Here's how the part is built. I have some questions about the finished solid (model axes, mm). A direction names the side the tool comes from. Give positions to 0.01 mm unless a question says otherwise; leave off trailing zeros. Loops run counter-clockwise (first coordinate to the right, second up) from the corner with the lowest first, then second, coordinate; pieces in that order, holes last.
Q1. If we section it at B-B (x = 10.5): Please give me the cut outline in (y, z), plus the area to 3 significant figures.
Q2. If we section it at C-C (z = 9): Please give me the cut outline in (x, y).
Q3. We'd pull the mould along Z, two halves only. Please class faces 4 (the face through (-13, 10, -28)), 5 (the face through (0.506, 9.86, 22.994)), 6 (the face through (13, 10, -19)): +Z half, -Z half, draft (parallel to the pull), parting line (faces both ways), or undercut.
Q4. I need wall thicknesses on line 1 (Y direction, x = -9.75, z = -22); line 2 (Z direction, x = 13, y = 11.75); line 3 (Z direction, x = -14, y = 8). Which ranges of each line are inside material? Lowest first, please.
Q5. If we section it at A-A (y = 10): Please give me the cut outline in (x, z).
Q6. Will these pins go through, and if not, where does the flat tip stop? P1, Ø3, axis at x = -0.5, y = 2, coming from the -Z side; P2, Ø4, axis at y = 4.5, z = 12, coming from the +X side; P3, Ø3, axis at x = -16, y = 9.5, coming from the +Z side; P4, Ø5, axis at y = 10, z = -22, coming from the +X side.
Q7. For faces 1 (the face through (-13, 7.5, -24.3)), 2 (the face through (-0.756, 9.86, 17.984)), 3 (the face through (-2.5, 9.9, -25.2)), which set-ups out of +Z, -Z, +X, -X, +Y, -Y let a thin tool reach every point of the face, with its end or its side?
Q8. If we section it at D-D (y = 18.25): Please give me the cut outline in (x, z), plus the area to 3 significant figures.
from build123d import *

# Parameters (mm, degrees)
BOSS_EXTRU_1_DEPTH      = 20
ESQUISSE2_R             = 3
ENL_V_MAT_EXTRU_1_DEPTH = 47
ENL_V_MAT_EXTRU_2_DEPTH = 10


with BuildPart() as part:
    # Esquisse1 → Boss.-Extru.1 (new body)
    with BuildSketch(Plane(origin=(0, 0, 0), x_dir=(1, 0, 0), z_dir=(0, 1, 0))):
        with BuildLine():
            Line((-23, 0), (-23, 28))
            Line((-23, 28), (-2.5, 28))
            Line((-2.5, 28), (-2.5, 17.82554347))
            ThreePointArc((-2.5, 17.82554347), (0, -18), (2.5, 17.82554347))
            Line((2.5, 17.82554347), (2.5, 28))
            Line((2.5, 28), (23, 28))
            Line((23, 28), (23, 0))
            ThreePointArc((23, 0), (0, -23), (-23, 0))
        make_face()
    extrude(amount=BOSS_EXTRU_1_DEPTH)

    # Esquisse2 → Enlèv. mat.-Extru.1 (cut, through all)
    with BuildSketch(Plane(origin=(23, 0, 0), x_dir=(0, 0, -1), z_dir=(1, 0, 0))):
        with Locations((22, 10)):
            Circle(ESQUISSE2_R)
    extrude(amount=-ENL_V_MAT_EXTRU_1_DEPTH, mode=Mode.SUBTRACT)

    # Esquisse3 → Enlèv. mat.-Extru.2 (cut)
    with BuildSketch(Plane.ZY.offset(23)):
        Polygon((-22, 4.226497308), (-17, 7.113248654), (-17, 12.886751346), (-22, 15.773502692), (-27, 12.886751346), (-27, 7.113248654), align=None)
    extrude(amount=-ENL_V_MAT_EXTRU_2_DEPTH, mode=Mode.SUBTRACT)


solid = part.part
Check sheet entries:
1. outline: (0, -28) - (20, -28) - (20, -14.62) - (0, -14.62) - close; (0, 14.62) - (20, 14.62) - (20, 20.46) - (0, 20.46) - close; hole circle Ø6 at (10, -22)
1. area: 356 mm2
2. outline: (-21.17, 0) - (-15.59, 0) - (-15.59, 20) - (-21.17, 20) - close; (15.59, 0) - (21.17, 0) - (21.17, 20) - (15.59, 20) - close
3. face 4: -Z half
3. face 5: +Z half
3. face 6: undercut
4. line 1: y = 0 to 7, 13 to 20
4. line 2: z = -28 to -24.44, -19.56 to -12.45, 12.45 to 18.97
4. line 3: z = -28 to -27, -17 to -11.31, 11.31 to 18.25
5. outline: (-23, -28) - (-2.5, -28) - (-2.5, -25) - (-13, -25) - (-13, -27) - (-23, -27) - close; (-23, -17) - (-13, -17) - (-13, -19) - (-2.5, -19) - (-2.5, -17.83) arc R18 cw (long way) to (2.5, -17.83) - (2.5, -19) - (23, -19) - (23, 0) arc R23 ccw to (-23, 0) - close; (2.5, -28) - (23, -28) - (23, -25) - (2.5, -25) - close
6. P1: stops at z = 17.89
6. P2: stops at x = 20.71
6. P3: stops at z = 17.85
6. P4: passes through
7. face 1: -X
7. face 2: +Y, -Y
7. face 3: -Z, +Y, -Y
8. outline: (-23, -28) - (-2.5, -28) - (-2.5, -17.83) arc R18 cw (long way) to (2.5, -17.83) - (2.5, -28) - (23, -28) - (23, 0) arc R23 ccw to (-23, 0) - close
8. area: 1,050 mm2
